Input: dimensioned drawing with shaded views. Units: mm. Origin: part minimum x, y, z. A direction names the side the tool comes from. Round coordinates to 2 decimals unless told otherwise and drop trailing zeros. Order: outer loops, then holes, each group sorted by start corner. A loop starts at its lowest first (then second) coordinate and runs counter-clockwise, first axis right, second up. Notation, with made-up numbers: (-9.75, 29.25) - (23.25, 29.25) arc R20 ccw to (23.25, 67.25) - close; hole circle Ø2 at (70, -7.5). An arc over 180 degrees is marked (long way). Return JSON: item names as keys, results as strings. Group by question number.
1) Access query for the marked faces 1 and 2. Directions: +Z, -Z, +X, -X, +Y, -Y. A direction counts if a zero-diameter tool reaches every point of the face in a straight line with its end or side. Return the directions, or none.
2) Contact query for flat-ended pins moving along their axis: P1, Ø12, axis at x = 28.5, z = 29, coming from the +Y side; P2, Ø1, axis at y = 10, z = 28.5, coming from the +X side. Output: stop coordinate, or through.
3) Ray query, line 1 (Y direction, x = 17.4, z = 6); line 2 (Y direction, x = 17.4, z = 20.25). Return the intervals inside material, ascending. Write a range as from..to.
4) Section B-B, the plane z = 50. Return loops of the section in (x, y), plus the area to 3 significant figures.
5) Section C-C, the plane z = 40. Return loops of the section in (x, y).
6) Section A-A, the plane z = 6. Return loops of the section in (x, y).
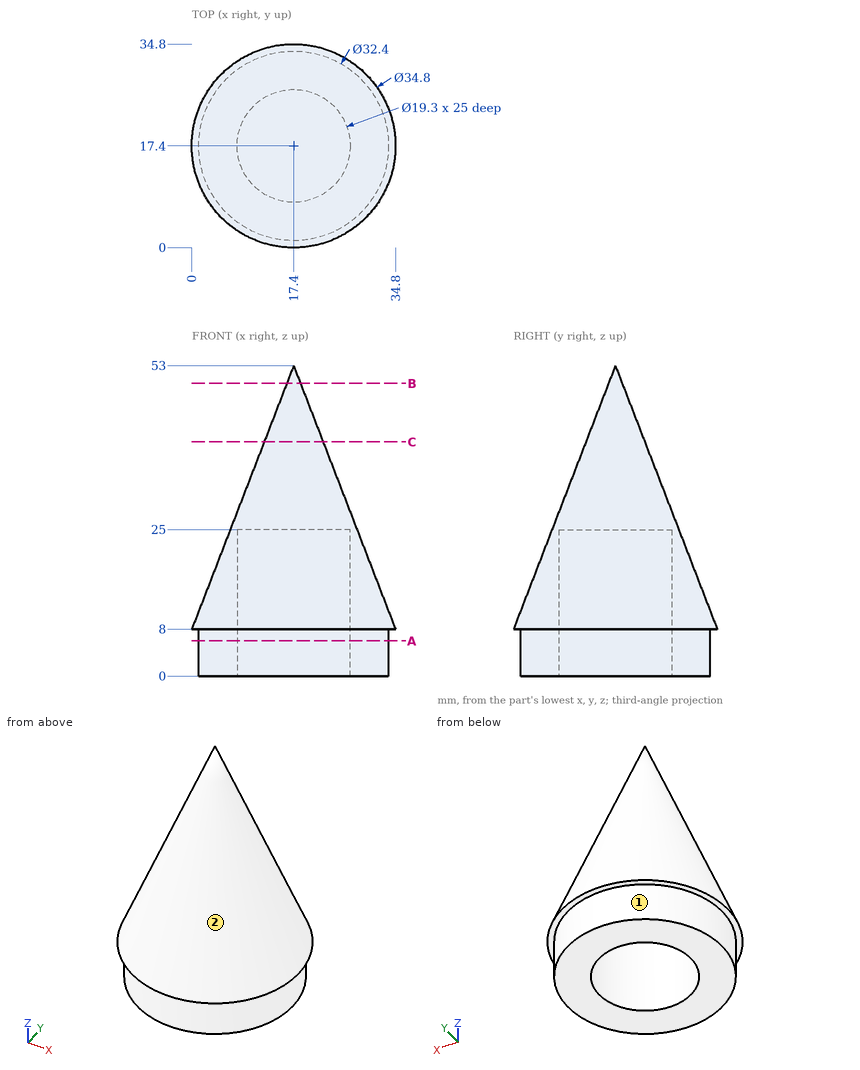
Geometry check:
{
 "1": {"face 1": "-Z", "face 2": "+Z"},
 "2": {"P1": "y = 26.02", "P2": "x = 23.96"},
 "3": {"line 1": "1.2..7.75, 27.05..33.6", "line 2": "4.74..7.75, 27.05..30.06"},
 "4": {"outline": "circle Ø2.32 at (17.4, 17.4)", "area": "4.23 mm2"},
 "5": {"outline": "circle Ø10.05 at (17.4, 17.4)"},
 "6": {"outline": "circle Ø32.4 at (17.4, 17.4); hole circle Ø19.3 at (17.4, 17.4)"}
}
